Job drawing, mm, ordinate dimensions from the low corner. One solid piece. Coordinates: 2 decimals unless noted, no trailing zeros. Order: outer loops, then holes, each group sorted by start corner. A loop starts at its lowest first (then second) coordinate and runs counter-clockwise, first axis right, second up. Notation, with made-up numbers: M 43,47.25 L 85,47.25 A32 cw 85,83.25 Z; hole C 37.5,17 d11. An arc over 180 degrees is marked long. Write item = value, one per line. Start each with the question number.
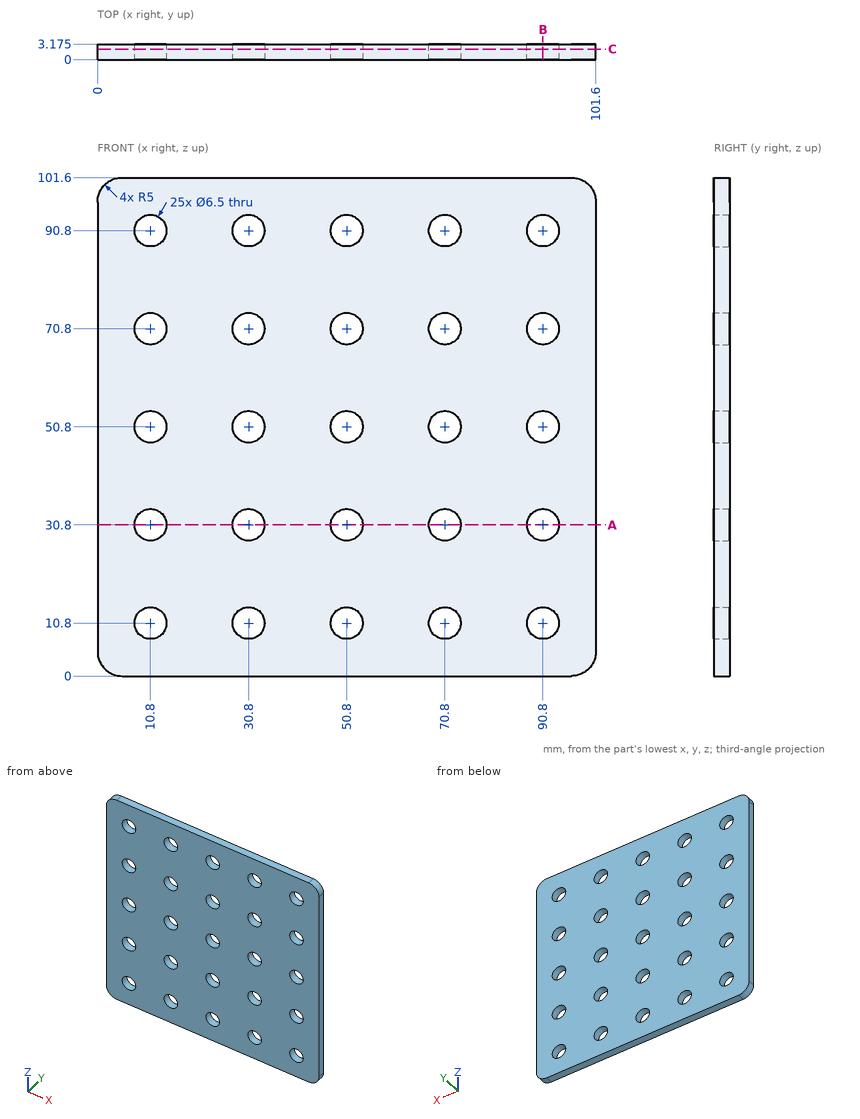
1. Slice it at B-B (x = 90.8). Write the cut outline in (y, z) (3 decimals), plus the area to 3 significant figures.
2. Slice it at C-C (y = 2.15). Give the number of separate pieces and of enclosed holes in the cut face, plus the area to 3 significant figures.
3. Probe L1, parallel to X at y = 2.25, z = 30.8; L2, parallel to Z at x = 71, y = 2.1; L3, parallel to Z at x = 88.5, y = 0.25. List the from-to ranges inside material, lowest first.
4. Flat gauge pins, fed straight in: pin 1 (6 mm diameter, centred on x = 30.8, z = 90.8, fed in from -Y); pin 2 (8 mm diameter, centred on x = 15, z = 16.5, fed in from -Y). Where does each tip first touch, or does it go through?
5. Slice it at A-A (z = 30.8). Write the cut outline in (x, y) (3 decimals).
Calculated:
q1.outline = M 0,0 L 3.175,0 L 3.175,7.55 L 0,7.55 Z; M 0,14.05 L 3.175,14.05 L 3.175,27.55 L 0,27.55 Z; M 0,34.05 L 3.175,34.05 L 3.175,47.55 L 0,47.55 Z; M 0,54.05 L 3.175,54.05 L 3.175,67.55 L 0,67.55 Z; M 0,74.05 L 3.175,74.05 L 3.175,87.55 L 0,87.55 Z; M 0,94.05 L 3.175,94.05 L 3.175,101.6 L 0,101.6 Z
q1.area = 219 mm²
q2.separate_pieces = 1
q2.enclosed_holes = 25
q2.area = 9,470 mm²
q3.L1 = 0 to 7.55, 14.05 to 27.55, 34.05 to 47.55, 54.05 to 67.55, 74.05 to 87.55, 94.05 to 101.6
q3.L2 = 0 to 7.56, 14.04 to 27.56, 34.04 to 47.56, 54.04 to 67.56, 74.04 to 87.56, 94.04 to 101.6
q3.L3 = 0 to 8.5, 13.1 to 28.5, 33.1 to 48.5, 53.1 to 68.5, 73.1 to 88.5, 93.1 to 101.6
q4.pin_1 = through
q4.pin_2 = 0
q5.outline = M 0,0 L 7.55,0 L 7.55,3.175 L 0,3.175 Z; M 14.05,0 L 27.55,0 L 27.55,3.175 L 14.05,3.175 Z; M 34.05,0 L 47.55,0 L 47.55,3.175 L 34.05,3.175 Z; M 54.05,0 L 67.55,0 L 67.55,3.175 L 54.05,3.175 Z; M 74.05,0 L 87.55,0 L 87.55,3.175 L 74.05,3.175 Z; M 94.05,0 L 101.6,0 L 101.6,3.175 L 94.05,3.175 Z
